CAD build for the part. Positions are in the model's coordinates, mm. A direction names the side the tool comes from. Give positions to 0.01 mm unless a question says otherwise; leave off trailing zeros. Order: outer loops, then holes, each group sorted by start corner. A loop starts at its lowest first (then second) coordinate and runs counter-clockwise, first axis right, second up.
```python
from build123d import *

# Parameters (mm, degrees)
SKETCH_1_R      = 4.5
SKETCH_1_R_2    = 1.35
EXTRUDE_1_DEPTH = 3
FILLET_1_R      = 10
FILLET_2_R      = 10


with BuildPart() as part:
    # 草图1 → 凸台-拉伸1 (new body)
    with BuildSketch(Plane(origin=(0, 0, 0), x_dir=(1, 0, 0), z_dir=(0, 1, 0))):
        with BuildLine():
            Line((-41.902581816, -0.567340904), (-10, -6.75))
            Line((-10, -6.75), (10, -6.75))
            Line((10, -6.75), (41.902581816, -0.567340904))
            ThreePointArc((41.902581816, -0.567340904), (45.340176894, 17.704733038), (30.317541634, 6.75))
            Line((30.317541634, 6.75), (-30.317541634, 6.75))
            ThreePointArc((-30.317541634, 6.75), (-45.340176894, 17.704733038), (-41.902581816, -0.567340904))
        make_face()
        with Locations(Location((-40, 9.25, 0), (0, 0, 270))):
            Circle(SKETCH_1_R, mode=Mode.SUBTRACT)
        with Locations(Location((-6, -4, 0), (0, 0, 270))):
            Circle(SKETCH_1_R_2, mode=Mode.SUBTRACT)
        with Locations(Location((-6, 4, 0), (0, 0, 270))):
            Circle(SKETCH_1_R_2, mode=Mode.SUBTRACT)
        with Locations(Location((6, -4, 0), (0, 0, 270))):
            Circle(SKETCH_1_R_2, mode=Mode.SUBTRACT)
        with Locations(Location((6, 4, 0), (0, 0, 270))):
            Circle(SKETCH_1_R_2, mode=Mode.SUBTRACT)
        with Locations(Location((40, 9.25, 0), (0, 0, 270))):
            Circle(SKETCH_1_R, mode=Mode.SUBTRACT)
    extrude(amount=EXTRUDE_1_DEPTH)

    # 圆角1
    fillet_1_edges = [part.edges().sort_by_distance(p)[0] for p in [
        (-30.317541634, 1.5, -6.75),
        (30.317541634, 1.5, -6.75),
    ]]
    fillet(fillet_1_edges, radius=FILLET_1_R)

    # 圆角2
    fillet_2_edges = [part.edges().sort_by_distance(p)[0] for p in [
        (10, 1.5, 6.75),
        (-10, 1.5, 6.75),
    ]]
    fillet(fillet_2_edges, radius=FILLET_2_R)


solid = part.part
```
Item 1: Slice it at A-A (x = -6). Give the cut face in (y, z), and give its area (3 significant figures).
Item 2: Slice it at B-B (y = 1.6). Give the cut face in (x, z).
Item 3: Two-plate mould, pull along Z, no slides. Class faces 3 (the face through (-1, 3, -4)), 4 (the face through (-10.009, 1.521, 6.703)), 5 (the face through (7.339, 1.479, -4.176)): released by +Z, released by -Z, zero draft, split by the parting line, or undercut.
Item 4: Slice it at D-D (z = -9.25). Give the cut face in (x, y), and give its area (3 significant figures).
Item 5: Wall check: L1, parallel to X at y = 2.15, z = -4; L2, parallel to Z at x = -37.5, y = 1.25; L3, parallel to X at y = 0.7, z = -13.25. Give the ranges that are in metal, low to high.
Item 6: Drop flat-ended pins along their axis: pin 1 Ø0.9 at (x, y) = (-3.5, 1) entering from -Z; pin 2 Ø1.5 at (x, y) = (35.5, 0.5) entering from +Z. Give the stop position or say it passes through.
Item 7: Slice it at C-C (z = 4). Give the cut face in (x, y), and give its area (3 significant figures).
Item 8: Tool access for faces 1 (the face through (0, 1, -6.75)), 2 (the face through (-1, 0, -4)): list every direction of +Z, -Z, +X, -X, +Y, -Y with a clear straight run to the whole face (end or side of a thin tool).
A:
1. outline: (0, -6.75) - (3, -6.75) - (3, -5.35) - (0, -5.35) - close; (0, -2.65) - (3, -2.65) - (3, 2.65) - (0, 2.65) - close; (0, 5.35) - (3, 5.35) - (3, 6.75) - (0, 6.75) - close
1. area: 24.3 mm2
2. outline: (-41.9, 0.57) arc R10 ccw (long way) to (-30.73, -13) arc R10 cw to (-21.46, -6.75) - (21.46, -6.75) arc R10 cw to (30.73, -13) arc R10 ccw (long way) to (41.9, 0.57) - (10.94, 6.57) arc R10 ccw to (9.04, 6.75) - (-9.04, 6.75) arc R10 ccw to (-10.94, 6.57) - close; hole circle Ø9 at (-40, -9.25); hole circle Ø2.7 at (-6, -4); hole circle Ø2.7 at (-6, 4); hole circle Ø2.7 at (6, -4); hole circle Ø2.7 at (6, 4); hole circle Ø9 at (40, -9.25)
3. face 3: zero draft
3. face 4: released by +Z
3. face 5: undercut
4. outline: (-50, 0) - (-44.5, 0) - (-44.5, 3) - (-50, 3) - close; (-35.5, 0) - (-28.07, 0) - (-28.07, 3) - (-35.5, 3) - close; (28.07, 0) - (35.5, 0) - (35.5, 3) - (28.07, 3) - close; (44.5, 0) - (50, 0) - (50, 3) - (44.5, 3) - close
4. area: 77.6 mm2
5. L1: x = -48.51 to -7.35, -4.65 to 4.65, 7.35 to 48.51
5. L2: z = -18.93 to -12.99, -5.51 to 1.42
5. L3: x = -49.17 to -42.06, -37.94 to -30.83, 30.83 to 37.94, 42.06 to 49.17
6. pin 1: stops at z = -6.75
6. pin 2: stops at z = 1.95
7. outline: (-24.19, 0) - (-7.35, 0) - (-7.35, 3) - (-24.19, 3) - close; (-4.65, 0) - (4.65, 0) - (4.65, 3) - (-4.65, 3) - close; (7.35, 0) - (24.19, 0) - (24.19, 3) - (7.35, 3) - close
7. area: 129 mm2
8. face 1: -Z, +Y, -Y
8. face 2: +Z, -Z, +X, -X, -Y
